Geometry: final body of the model. Coordinates: model frame, mm. Give positions to 0.01 mm unless a question says otherwise; leave off trailing zeros. Order: outer loops, then holes, each group sorted by start corner. A loop starts at its lowest first (then second) coordinate and runs counter-clockwise, first axis right, second up. Notation, with made-up numbers: (31, -9.5) -> (71, -9.5) arc R14 cw to (71, 4.5) -> close; hole circle Ø8 at (30.25, -24). An arc over 180 degrees is marked (long way). One line per question, with ' | ' between items.
from build123d import *

# Parameters (mm, degrees)
F0_W     = 76.2
F0_H     = 127
F1_DEPTH = 2
F3_DEPTH = 25


with BuildPart() as f1:
    # F0 (on Top) → F1 (new body)
    with BuildSketch(Plane.XY):
        Rectangle(F0_W, F0_H)
    extrude(amount=F1_DEPTH)

    # F2 (on face) → F3 (cut)
    with BuildSketch(Plane.XY.offset(2)):
        with BuildLine():
            Line((38.1, 63.5), (10, 63.5))
            Line((10, 63.5), (19.592162, 27.701563))
            ThreePointArc((19.592162, 27.701563), (26.43569, 17.4595), (38.1, 13.5))
            Line((38.1, 13.5), (38.1, 63.5))
        make_face()
    extrude(amount=-F3_DEPTH, mode=Mode.SUBTRACT)


solid = f1.part
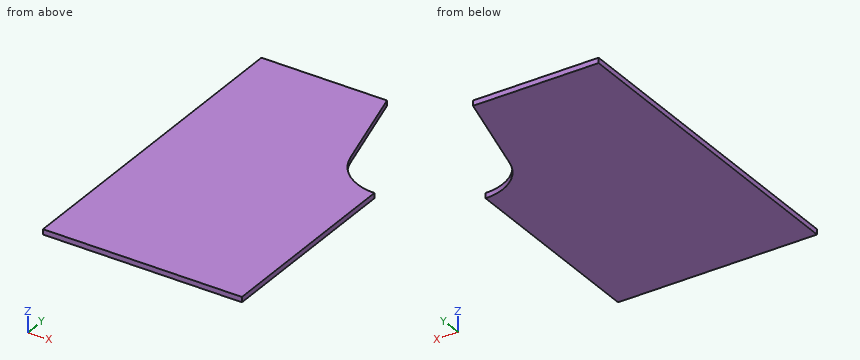
1) Section A-A on z = 1.45. Return loops of the section in (x, y), plus the area to 3 significant figures.
Check result:
outline: (-38.1, -63.5) -> (38.1, -63.5) -> (38.1, 13.5) arc R19.16 cw to (19.59, 27.7) -> (10, 63.5) -> (-38.1, 63.5) -> close | area: 8,650 mm^2
2) Section C-C on x = 33. Return loops of the section in (y, z), plus the area to 3 significant figures.
Check result:
outline: (-63.5, 0) -> (14.19, 0) -> (14.19, 2) -> (-63.5, 2) -> close | area: 155 mm^2
3) Material intervals for probe 1 along X at (y, z) = (51.5, 0.2); probe 2 along X at (y, z) = (26, 1.75); probe 3 along Y at (x, z) = (27.5, 0.9), sorted ascending. Write a range as from..to.
Check result:
probe 1: x = -38.1..13.22 | probe 2: x = -38.1..20.13 | probe 3: y = -63.5..16.7
4) Section B-B on y = 42. Return loops of the section in (x, z), plus the area to 3 significant figures.
Check result:
outline: (-38.1, 0) -> (15.76, 0) -> (15.76, 2) -> (-38.1, 2) -> close | area: 108 mm^2
